Can you work these out from the drawing? Everything is in mm from the part's minimum corner. A direction names the side the tool comes from. Coordinates: 2 decimals unless noted, no trailing zeros. Loops run counter-clockwise (first coordinate to the right, second up) from the corner with the lowest first, then second, coordinate; pieces in that order, holes last. Notation, with made-up numbers: (-20, 3) -> (30, 3) arc R15 ccw to (30, 30) -> close; hole circle Ø3 at (-0.75, 21.5). An arc over 180 degrees is marked (long way). Put each result on its own line as item: value. Start each with the question number.
Item 1: Will these pins go through, and if not, where does the flat tip stop? P1, Ø5, axis at x = 54, z = 247.5, coming from the +Y side; P2, Ø12, axis at y = 28.5, z = 100, coming from the -X side; P3, Ø12.5, axis at x = 52, z = 145.5, coming from the -Y side; P4, Ø3, axis at x = 40, z = 220.5, coming from the -Y side.
Item 2: If we section it at A-A on y = 20: Please give me the cut outline in (x, z).
Item 3: For the marked faces 1 and 2, which set-ups out of +Z, -Z, +X, -X, +Y, -Y let a thin tool reach every point of the face, with its end or its side?
Item 4: Please list where these lines run through material, in increasing order: L1, parallel to X at y = 7, z = 260.5; L2, parallel to X at y = 20, z = 239. Write a range as from..to.
Item 5: If we section it at C-C on z = 57: Please give me the cut outline in (x, y), plus the area to 3 significant figures.
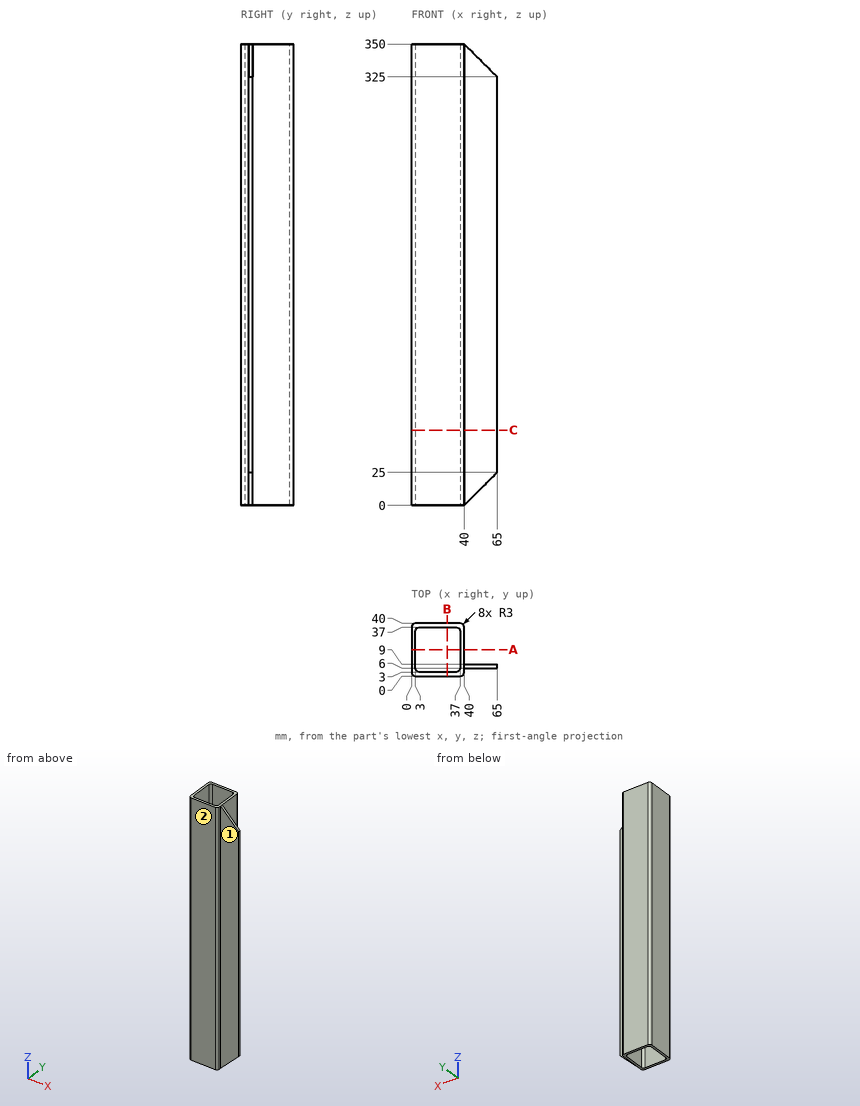
Solutions:
1. P1: y = 9
1. P2: x = 0
1. P3: y = 6
1. P4: y = 0.4
2. outline: (0, 0) -> (3, 0) -> (3, 350) -> (0, 350) -> close; (37, 0) -> (40, 0) -> (40, 350) -> (37, 350) -> close
3. face 1: +Z, -Z, +X, -Y
3. face 2: +Z, -Z, +X, -X, -Y
4. L1: 0..3, 37..65
4. L2: 0..3, 37..40
5. outline: (0, 3) arc R3 ccw to (3, 0) -> (37, 0) arc R3 ccw to (40, 3) -> (40, 6) -> (65, 6) -> (65, 9) -> (40, 9) -> (40, 37) arc R3 ccw to (37, 40) -> (3, 40) arc R3 ccw to (0, 37) -> close; hole (3, 6) arc R3 ccw to (6, 3) -> (34, 3) arc R3 ccw to (37, 6) -> (37, 34) arc R3 ccw to (34, 37) -> (6, 37) arc R3 ccw to (3, 34) -> close
5. area: 519 mm^2
